from build123d import *

# Parameters (mm, degrees)
SKETCH1_W           = 22.5
SKETCH1_H           = 16.5
BOSS_EXTRUDE1_DEPTH = 9
SKETCH3_W           = 14.5
SKETCH3_H           = 14.5
CUT_EXTRUDE2_DEPTH  = 74.330139174
DRAFT1_ANGLE        = 16
DRAFT3_ANGLE        = 16
SKETCH9_W           = 3
SKETCH9_H           = 3
CUT_EXTRUDE3_DEPTH  = 14.5


with BuildPart() as part:
    # Sketch1 → Boss-Extrude1 (new body)
    with BuildSketch(Plane(origin=(0, 0, 0), x_dir=(1, 0, 0), z_dir=(0, 1, 0))):
        with Locations((-33.839285714, -48.875)):
            Rectangle(SKETCH1_W, SKETCH1_H)
    extrude(amount=BOSS_EXTRUDE1_DEPTH)

    # Sketch3 → Cut-Extrude2 (cut, through all)
    with BuildSketch(Plane.XZ):
        with Locations((-33.839285714, 47.875)):
            Rectangle(SKETCH3_W, SKETCH3_H)
    extrude(amount=-CUT_EXTRUDE2_DEPTH, mode=Mode.SUBTRACT)

    # Draft1
    draft1_faces = [part.faces().sort_by_distance(p)[0] for p in [
        (-45.089285714, 4.5, 48.875),
    ]]
    draft(draft1_faces, Plane(origin=(0, 0, 0), x_dir=(0, 0, -1), z_dir=(0, -1, 0)), DRAFT1_ANGLE)

    # Draft3
    draft3_faces = [part.faces().sort_by_distance(p)[0] for p in [
        (-34.496127322, 4.58135782, 57.125),
    ]]
    draft(draft3_faces, Plane(origin=(0, 0, 0), x_dir=(0, 0, -1), z_dir=(0, -1, 0)), DRAFT3_ANGLE)

    # Sketch9 → Cut-Extrude3 (cut)
    with BuildSketch(Plane(origin=(0, 0, 40.625), x_dir=(-1, 0, 0), z_dir=(0, 0, 1))):
        with Locations((25.089285714, -3.5)):
            Rectangle(SKETCH9_W, SKETCH9_H)
        with Locations((42.589285714, -3.5)):
            Rectangle(SKETCH9_W, SKETCH9_H)
    extrude(amount=CUT_EXTRUDE3_DEPTH, mode=Mode.SUBTRACT)


solid = part.part
For this review, take the finished solid that the model builds, in its own axes (mm). A direction names the side the tool comes from. Round coordinates to 2 decimals unless told otherwise and drop trailing zeros. Loops run counter-clockwise (first coordinate to the right, second up) from the corner with the lowest first, then second, coordinate; pieces in that order, holes last. Notation, with made-up numbers: (64, -15) - (81, -15) arc R17 ccw to (81, 11) - close; hole circle Ø11 at (79, -3.5). An arc over 180 degrees is marked (long way). Use one line per item in the form item = value.
Item 1: Consider section B-B on x = -25.5. Write out the cut boundary in (y, z) (3 decimals), then the cut area to 3 significant figures.
Answers:
outline = (0, 40.625) - (2, 40.625) - (2, 55.125) - (5, 55.125) - (5, 40.625) - (9, 40.625) - (9, 59.706) - (0, 57.125) - close
area = 117 mm^2
Item 2: Consider section C-C on y = 4. Write out the cut boundary in (x, z) (3 decimals).
Answers:
outline = (-46.236, 40.625) - (-44.089, 40.625) - (-44.089, 55.125) - (-23.589, 55.125) - (-23.589, 40.625) - (-22.589, 40.625) - (-22.589, 58.272) - (-46.236, 58.272) - close
Item 3: Mouldability with a two-part tool opening along X and no side actions: class faces 1 (the flat face through (-22.589, 4, 50)), 2 (the flat face through (-46.362, 4.437, 50.299)), 3 (the flat face through (-34, 4, 55.125)), 4 (the flat face through (-26.589, 1, 48)) as +X half, -X half, draft (parallel to the pull), parting line (faces both ways), or undercut.
Answers:
face_1 = +X half
face_2 = -X half
face_3 = undercut
face_4 = undercut
Item 4: Consider section D-D on z = 55.75. Write out the cut boundary in (x, y), then the cut area to 3 significant figures.
Answers:
outline = (-47.67, 9) - (-45.09, 0) - (-22.59, 0) - (-22.59, 9) - close
area = 214 mm^2
Item 5: Consider section A-A on z = 44.5. Write out the cut boundary in (x, y), then the cut area to 3 significant figures.
Answers:
outline = (-47.67, 9) - (-45.09, 0) - (-41.09, 0) - (-41.09, 2) - (-44.09, 2) - (-44.09, 5) - (-41.09, 5) - (-41.09, 9) - close; (-26.59, 0) - (-22.59, 0) - (-22.59, 9) - (-26.59, 9) - (-26.59, 5) - (-23.59, 5) - (-23.59, 2) - (-26.59, 2) - close
area = 65.6 mm^2
Item 6: Clearance check with flat-ended pins moving along their axes: P1, Ø4, axis at x = -41, y = 5.5, coming from the +Z side; P2, Ø1, axis at x = -43, y = 7.5, coming from the +Z side; P3, Ø1.5, axis at y = 7.5, z = 49.5, coming from the -X side. State where each tip first meets the part, or that it passes through.
Answers:
P1 = 59.28
P2 = 59.42
P3 = -47.45
Item 7: For line 1 (Y direction, x = -42.5, z = 53.5); line 2 (X direction, y = 7.25, z = 42.25); line 3 (X direction, y = 6.25, z = 47.25), list the stretches that pass through material, from the lowest coordinate up.
Answers:
line_1 = 0 to 2, 5 to 9
line_2 = -47.17 to -41.09, -26.59 to -22.59
line_3 = -46.88 to -41.09, -26.59 to -22.59
Item 8: Tool access review of faces 5 (the flat face through (-23.589, 4, 48)), 6 (the flat face through (-41.089, 1, 48)), 7 (the flat face through (-38, 9, 56)): name each direction out of +Z, -Z, +X, -X, +Y, -Y from which nothing blocks a thin tool from reaching the whole face with its end or side.
Answers:
face_5 = -Z
face_6 = -Z, +Y, -Y
face_7 = +Z, -Z, +X, -X, +Y
